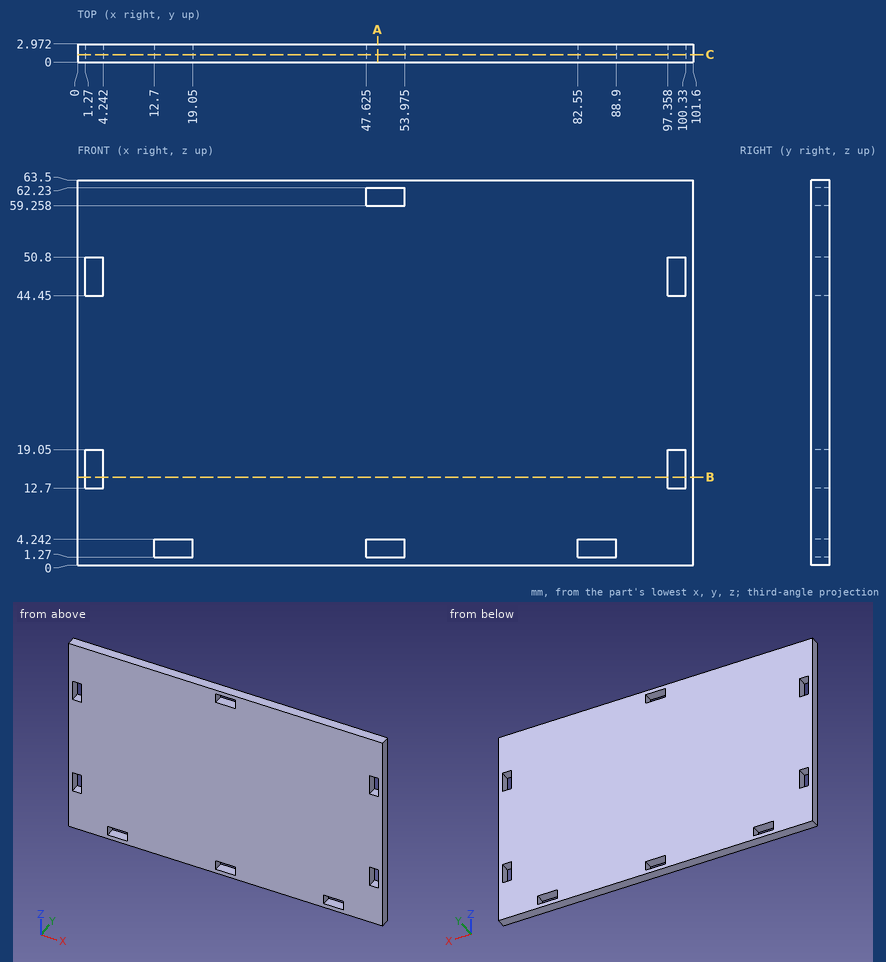
The figure shows three views and two pictorial views of one solid part (mm, origin at its lowest corner). Answer the questions. Coordinates: 2 decimals unless noted, no trailing zeros. Loops run counter-clockwise (first coordinate to the right, second up) from the corner with the lowest first, then second, coordinate; pieces in that order, holes last. Notation, with made-up numbers: (2, 37) -> (19, 37) arc R15 ccw to (19, 41) -> close; hole circle Ø4 at (-35, 78). An arc over 180 degrees is marked (long way). Return JSON: item names as keys, results as strings. Group by question number.
(1) A cutting plane is placed at A-A on x = 49.5. Write down the section's boundary in (y, z).
(2) A cutting plane is placed at C-C on y = 1.2. Count the separate pieces of the cut face and the enclosed holes in it, and give its area (3 significant figures).
(3) A cutting plane is placed at B-B on z = 14.5. Write down the section's boundary in (x, y).
(4) Find the intervals of material crossed by probe 1 along Z at (x, y) = (4, 2); probe 2 along X at (y, z) = (1.6, 3) (3 decimals); probe 3 along X at (y, z) = (0.65, 44.5), in increasing order. Write a range as from..to.
The answers:
{
 "1": {"outline": "(0, 0) -> (2.97, 0) -> (2.97, 1.27) -> (0, 1.27) -> close; (0, 4.24) -> (2.97, 4.24) -> (2.97, 59.26) -> (0, 59.26) -> close; (0, 62.23) -> (2.97, 62.23) -> (2.97, 63.5) -> (0, 63.5) -> close"},
 "2": {"separate pieces": "1", "enclosed holes": "8", "area": "6,300 mm^2"},
 "3": {"outline": "(0, 0) -> (1.27, 0) -> (1.27, 2.97) -> (0, 2.97) -> close; (4.24, 0) -> (97.36, 0) -> (97.36, 2.97) -> (4.24, 2.97) -> close; (100.33, 0) -> (101.6, 0) -> (101.6, 2.97) -> (100.33, 2.97) -> close"},
 "4": {"probe 1": "z = 0..12.7, 19.05..44.45, 50.8..63.5", "probe 2": "x = 0..12.7, 19.05..47.625, 53.975..82.55, 88.9..101.6", "probe 3": "x = 0..1.27, 4.24..97.36, 100.33..101.6"}
}
